```python
from build123d import *

# Parameters (mm, degrees)
F0_W     = 63.5
F0_H     = 38.1
F1_DEPTH = 3.175
F2_W     = 22.225
F2_H     = 38.1
F2_W_2   = 3.175
F3_DEPTH = 3.175
F5_DEPTH = 76.2
F6_W     = 63.5
F6_H     = 114.3
F6_W_2   = 3.175
F7_DEPTH = 3.175
F8_W     = 63.5
F8_H     = 22.225
F9_DEPTH = 3.175


with BuildPart() as f1:
    # F0 (on Front) → F1 (new body)
    with BuildSketch(Plane.XZ):
        Rectangle(F0_W, F0_H)
    extrude(amount=F1_DEPTH)

    # F2 (on face) → F3 (join)
    with BuildSketch(Plane.YZ.offset(31.75)):
        with Locations((11.1125, 0)):
            Rectangle(F2_W, F2_H)
        with Locations((-1.5875, 0)):
            Rectangle(F2_W_2, F2_H)
    extrude(amount=F3_DEPTH)

    # F4 (on face) → F5 (join)
    with BuildSketch(Plane(origin=(0, 0, -19.05), x_dir=(1, 0, 0), z_dir=(0, 0, -1))):
        Polygon((31.75, -22.225), (34.925, -22.225), (34.925, 3.175), (31.75, 3.175), (31.75, 0), align=None)
    extrude(amount=F5_DEPTH)

    # F6 (on face) → F7 (join)
    with BuildSketch(Plane(origin=(0, 22.225, 0), x_dir=(-1, 0, 0), z_dir=(0, 1, 0))):
        with Locations((0, -38.1)):
            Rectangle(F6_W, F6_H)
        with Locations((-33.3375, -38.1)):
            Rectangle(F6_W_2, F6_H)
    extrude(amount=F7_DEPTH)

    # F8 (on face) → F9 (join)
    with BuildSketch(Plane.XY.offset(19.05)):
        with Locations((0, 11.1125)):
            Rectangle(F8_W, F8_H)
    extrude(amount=-F9_DEPTH)


solid = f1.part
```
Model file for the job. Use its own axes, mm. A direction names the side the tool comes from. Coordinates: 2 decimals unless noted, no trailing zeros. Order: outer loops, then holes, each group sorted by start corner. A loop starts at its lowest first (then second) coordinate and runs counter-clockwise, first axis right, second up. Notation, with made-up numbers: (49, -22) -> (71, -22) arc R11 cw to (71, -14) -> close; hole circle Ø11 at (62, -40). An arc over 180 degrees is marked (long way). Answer as a JSON object with one key per item and string values. Group by question number.
1) Which spindle directions (+Z, -Z, +X, -X, +Y, -Y) get a long thin tool onto all of the face, cutting with end or side? Do faces 5 (the face through (1, 11, 19.05)), 6 (the face through (0, 0, -1)). Say none if no direction does.
2) Pull direction Y, two halves, no side cores. Call faces 1 (the face through (0, -2, -19.05)), 2 (the face through (2, 25.4, -37)), 3 (the face through (0, 22.225, -39)), 4 (the face through (0, 11, 15.875)): +Y half, -Y half, draft (parallel to the pull), parting line (faces both ways), or undercut.
3) Cut at D-D, the plane z = -42. Write the cut outline in (x, y) (3 decimals).
4) Cut at C-C, the plane y = 6. Write the cut outline in (x, z) (3 decimals).
5) Cut at B-B, the plane x = 30. Write the cut outline in (y, z) (3 decimals).
6) Flat gauge pins, fed straight in: pin 1 (5 mm diameter, centred on y = 5, z = -32.5, fed in from -X); pin 2 (1.6 mm diameter, centred on x = 3, y = -1, fed in from -Z); pin 3 (4 mm diameter, centred on x = 13, y = 11.5, fed in from -Z) (3 decimals). Where does each tip first touch, or does it go through?
7) Drill centre lines: L1, parallel to Y at x = -14, z = -16.5 (3 decimals); L2, parallel to Z at x = 15, y = 20.5 (3 decimals); L3, parallel to X at y = 18.75, z = -56 (3 decimals). Where is each one in solid material? Low to high.
8) Cut at A-A, the plane z = 9.5. Write the cut outline in (x, y) (3 decimals), then the cut area to 3 significant figures.
Check values:
{
 "1": {"face 5": "+Z, +X, -X, +Y, -Y", "face 6": "-Z, -X"},
 "2": {"face 1": "draft", "face 2": "+Y half", "face 3": "undercut", "face 4": "undercut"},
 "3": {"outline": "(-31.75, 22.225) -> (31.75, 22.225) -> (31.75, -3.175) -> (34.925, -3.175) -> (34.925, 25.4) -> (-31.75, 25.4) -> close"},
 "4": {"outline": "(-31.75, 15.875) -> (31.75, 15.875) -> (31.75, -95.25) -> (34.925, -95.25) -> (34.925, 19.05) -> (-31.75, 19.05) -> close"},
 "5": {"outline": "(-3.175, -19.05) -> (0, -19.05) -> (0, 15.875) -> (22.225, 15.875) -> (22.225, -95.25) -> (25.4, -95.25) -> (25.4, 19.05) -> (-3.175, 19.05) -> close"},
 "6": {"pin 1": "stops at x = 31.75", "pin 2": "stops at z = -19.05", "pin 3": "stops at z = 15.875"},
 "7": {"L1": "y = -3.175 to 0, 22.225 to 25.4", "L2": "z = 15.875 to 19.05", "L3": "x = 31.75 to 34.925"},
 "8": {"outline": "(-31.75, -3.175) -> (34.925, -3.175) -> (34.925, 25.4) -> (-31.75, 25.4) -> (-31.75, 22.225) -> (31.75, 22.225) -> (31.75, 0) -> (-31.75, 0) -> close", "area": "494 mm²"}
}
